Study the drawing (mm; zero at the part's minimum x, y, z) and answer. A direction names the side the tool comes from. Coordinates: 2 decimals unless noted, no trailing zeros. Write each loop counter-clockwise with the first axis right and the second up, starting at its lowest first coordinate (ties: lowest second). Pieces come first, ordered by that corner, then holes. Notation, with made-up numbers: M 31,0.5 L 46,0.5 A19 cw 46,13.5 Z; hole C 64,76.5 d5. An arc over 180 degrees is marked long. Answer as a JSON object with one key per item and string values. Group by question number.
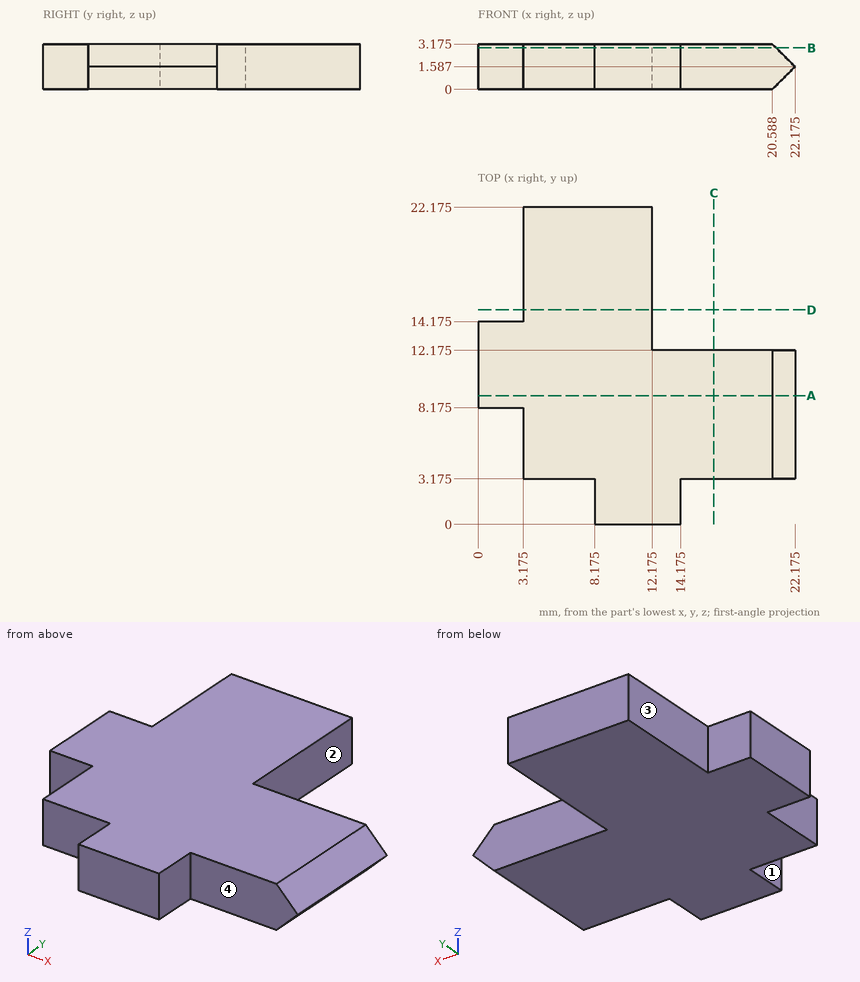
Item 1: A cutting plane is placed at B-B, the plane z = 2.9. Write down the section's boundary in (x, y) (1 decimal), and give its area (3 significant figures).
Item 2: A cutting plane is placed at C-C, the plane x = 16.5. Write down the section's boundary in (y, z) (1 decimal), and give its area (3 significant figures).
Item 3: Flat-ended cylindrical pins translate along their axes: pin 1 Ø1 at (y, z) = (1.5, 2) entering from +X (1 decimal); pin 2 Ø1 at (y, z) = (1.5, 2) entering from -X (1 decimal); pin 3 Ø1.5 at (x, y) = (4, 7) entering from -Z; pin 4 Ø1.6 at (x, z) = (17, 2.5) entering from +Y (1 decimal). Find the tip coordinate at first contact, or state that the pin passes through.
Item 4: A cutting plane is placed at A-A, the plane y = 9. Write down the section's boundary in (x, z) (1 decimal).
Item 5: A tool of negligible diameter and unlimited length cuts with its end or side. For the marked faces 1, 2, 3 and 4, from which of +Z, -Z, +X, -X, +Y, -Y can it reach the whole face along a straight path? Write none if from no direction.
Item 6: Consider L1, parallel to Y at x = 7.75, z = 2.65 (1 decimal); L2, parallel to X at y = 14.5, z = 1.4 (1 decimal); L3, parallel to Y at x = 13.5, z = 1.75 (1 decimal). Determine where each line is inside the solid, lowest interval first. Write a range as from..to.
Answer:
{
 "1": {"outline": "M 0,8.2 L 3.2,8.2 L 3.2,3.2 L 8.2,3.2 L 8.2,0 L 14.2,0 L 14.2,3.2 L 20.9,3.2 L 20.9,12.2 L 12.2,12.2 L 12.2,22.2 L 3.2,22.2 L 3.2,14.2 L 0,14.2 Z", "area": "287 mm2"},
 "2": {"outline": "M 3.2,0 L 12.2,0 L 12.2,3.2 L 3.2,3.2 Z", "area": "28.6 mm2"},
 "3": {"pin 1": "x = 14.2", "pin 2": "x = 8.2", "pin 3": "z = 0", "pin 4": "y = 12.2"},
 "4": {"outline": "M 0,0 L 20.6,0 L 22.2,1.6 L 20.6,3.2 L 0,3.2 Z"},
 "5": {"face 1": "+Z, -Z, -X, -Y", "face 2": "+Z, -Z, +X, +Y", "face 3": "+Z, -Z, -X, +Y", "face 4": "+Z, -Z, +X, -Y"},
 "6": {"L1": "3.2..22.2", "L2": "3.2..12.2", "L3": "0..12.2"}
}
